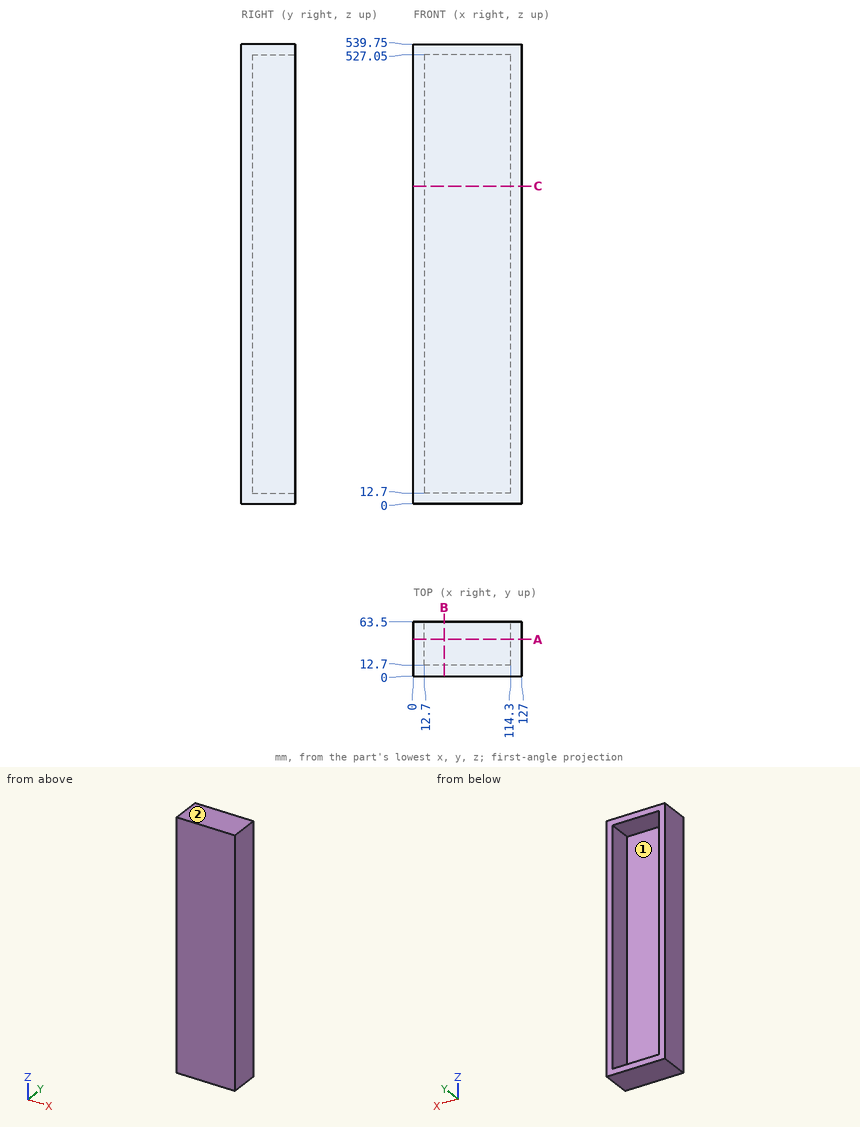
Input: dimensioned drawing with shaded views. Units: mm. Origin: part minimum x, y, z. A direction names the side the tool comes from. Give positions to 0.01 mm unless a question says otherwise; leave off trailing zeros. Order: outer loops, then holes, each group sorted by start corner. A loop starts at its lowest first (then second) coordinate and runs counter-clockwise, first axis right, second up.
(1) Material intervals for line 1 along Z through (x, y) = (90.5, 59.5); line 2 along X through (y, z) = (57, 101.5); line 3 along Y through (x, z) = (109, 287.5), sorted ascending.
(2) Section query B-B (x = 36). Return the cut outline in (y, z), plus the area to 3 significant figures.
(3) Contact query for flat-ended pins moving along their axis: P1, Ø8, axis at x = 24, z = 67, coming from the +Y side; P2, Ø5, axis at y = 33.5, z = 105.5, coming from the -X side. Output: stop coordinate, or through.
(4) Section query C-C (z = 373). Return the cut outline in (x, y), plus the area to 3 significant figures.
(5) Access query for the marked faces 1 and 2. Directions: +Z, -Z, +X, -X, +Y, -Y. A direction counts if a zero-diameter tool reaches every point of the face in a straight line with its end or side. Return the directions, or none.
(6) Section query A-A (y = 43). Return the cut outline in (x, z), plus the area to 3 significant figures.
Outcome:
1. line 1: z = 0 to 12.7, 527.05 to 539.75
1. line 2: x = 0 to 12.7, 114.3 to 127
1. line 3: y = 0 to 12.7
2. outline: (0, 0) - (63.5, 0) - (63.5, 12.7) - (12.7, 12.7) - (12.7, 527.05) - (63.5, 527.05) - (63.5, 539.75) - (0, 539.75) - close
2. area: 8,150 mm2
3. P1: stops at y = 12.7
3. P2: stops at x = 0
4. outline: (0, 0) - (127, 0) - (127, 63.5) - (114.3, 63.5) - (114.3, 12.7) - (12.7, 12.7) - (12.7, 63.5) - (0, 63.5) - close
4. area: 2,900 mm2
5. face 1: +Y
5. face 2: +Z, +X, -X, +Y, -Y
6. outline: (0, 0) - (127, 0) - (127, 539.75) - (0, 539.75) - close; hole (12.7, 12.7) - (114.3, 12.7) - (114.3, 527.05) - (12.7, 527.05) - close
6. area: 16,300 mm2
